Design review of the part built by this model. Coordinates are the model's own, in mm. Face numbers are marked on the shaded views. Coordinates: 2 decimals unless noted, no trailing zeros. Order: outer loops, then holes, each group sorted by start corner. A loop starts at its lowest first (then second) coordinate and runs counter-clockwise, first axis right, second up. Notation, with made-up numbers: M -24,-25.75 L -9,-25.75 A15 cw -9,-21.75 Z; hole C 82,69 d2. An arc over 180 degrees is marked long. Use CSV: the item, a comma, the result in double quotes.
```python
from build123d import *

# Parameters (mm, degrees)
SKETCH1_R           = 9.5
BOSS_EXTRUDE1_DEPTH = 25
SKETCH2_R           = 2.5
CUT_EXTRUDE1_DEPTH  = 15
SKETCH3_R           = 4
CUT_EXTRUDE2_DEPTH  = 20.767397401
CHAMFER1_SIZE       = 2
CUT_EXTRUDE3_REACH  = 34.806
SKETCH13_R          = 1


with BuildPart() as part:
    # Sketch1 → Boss-Extrude1 (new body)
    with BuildSketch(Plane(origin=(0, 0, 0), x_dir=(1, 0, 0), z_dir=(0, 1, 0))):
        with Locations(Location((0, 0, 0), (0, 0, 270))):
            Circle(SKETCH1_R)
    extrude(amount=BOSS_EXTRUDE1_DEPTH)

    # Sketch2 → Cut-Extrude1 (cut)
    with BuildSketch(Plane(origin=(0, 0, 0), x_dir=(1, 0, 0), z_dir=(0, 1, 0))):
        with Locations(Location((0, 0, 0), (0, 0, 270))):
            Circle(SKETCH2_R)
    extrude(amount=CUT_EXTRUDE1_DEPTH, mode=Mode.SUBTRACT)

    # Sketch3 → Cut-Extrude2 (cut, through all)
    with BuildSketch(Plane(origin=(0, 14.5, 0), x_dir=(1, 0, 0), z_dir=(0, 1, 0))):
        with Locations(Location((0, 0, 0), (0, 0, 90))):
            Circle(SKETCH3_R)
    extrude(amount=CUT_EXTRUDE2_DEPTH, mode=Mode.SUBTRACT)

    # Chamfer1
    chamfer1_edges = [part.edges().sort_by_distance(p)[0] for p in [
        (0, 0, -9.5),
        (0, 25, -9.5),
    ]]
    chamfer(chamfer1_edges, length=CHAMFER1_SIZE)

    # Sketch13 → Cut-Extrude3 (cut, up to next)
    with BuildSketch(Plane.XY.offset(9.5), mode=Mode.PRIVATE) as cut_extrude3_sk1:
        with Locations((0, 19)):
            Circle(SKETCH13_R)
    cut_extrude3_tool1 = extrude(cut_extrude3_sk1.sketch, amount=-CUT_EXTRUDE3_REACH, mode=Mode.PRIVATE) & part.part
    # Sketch13 → Cut-Extrude3 (cut, up to next)
    with BuildSketch(Plane.XY.offset(9.5), mode=Mode.PRIVATE) as cut_extrude3_sk2:
        with Locations((0, 7)):
            Circle(SKETCH13_R)
    cut_extrude3_tool2 = extrude(cut_extrude3_sk2.sketch, amount=-CUT_EXTRUDE3_REACH, mode=Mode.PRIVATE) & part.part
    add(cut_extrude3_tool1.solids().sort_by_distance((0, 19, 9.5))[0], mode=Mode.SUBTRACT)
    add(cut_extrude3_tool2.solids().sort_by_distance((0, 7, 9.5))[0], mode=Mode.SUBTRACT)


solid = part.part
```
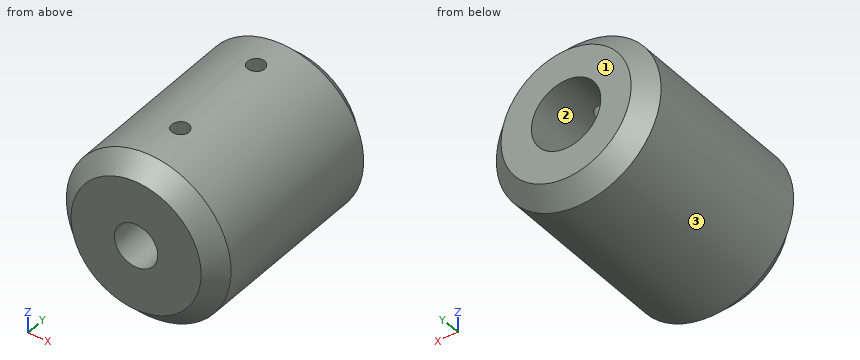
(1) The part is to be moulded in two halves that separate along Z. For the marked faces 1, 2 and 3, say which applies: pulls with the +Z half, pulls with the -Z half, needs draft (parallel to the pull), parting line crosses it, or undercut.
The answers:
face 1,"needs draft"
face 2,"undercut"
face 3,"parting line crosses it"
(2) Add section C-C on y = 21.75. State the section outline as (x, z) points.
The answers:
outline,"C 0,0 d19; hole C 0,0 d8"
(3) Add section D-D on y = 19. State the section outline as (x, z) points.
The answers:
outline,"M -1,3.87 L -1,9.45 A9.5 ccw long 1,9.45 L 1,3.87 A4 cw long Z"
(4) Add section B-B on z = 0. State the section outline as (x, y) points, and give its area (4 significant figures).
The answers:
outline,"M -9.5,2 L -7.5,0 L -2.5,0 L -2.5,14.5 L -4,14.5 L -4,25 L -7.5,25 L -9.5,23 Z; M 2.5,0 L 7.5,0 L 9.5,2 L 9.5,23 L 7.5,25 L 4,25 L 4,14.5 L 2.5,14.5 Z"
area,"310.5 mm2"
(5) Wall thickness on probe 1 along Y at (x, z) = (0, 4.5); probe 2 along X at (y, z) = (3.5, 0); probe 3 along X at (y, z) = (20.75, 0): over which ranges is each line inside the solid? List them lowest first.
The answers:
probe 1,"y = 0 to 6, 8 to 18, 20 to 25"
probe 2,"x = -9.5 to -2.5, 2.5 to 9.5"
probe 3,"x = -9.5 to -4, 4 to 9.5"
(6) Clearance check with flat-ended pins moving along their axes: P1, Ø2, axis at x = -2.5, y = 15, coming from the -Z side; P2, Ø1.6, axis at x = 0, y = 7, coming from the +Z side; P3, Ø1.8, axis at x = 0, y = 19, coming from the +Z side. State where each tip first meets the part, or that it passes through.
The answers:
P1,"stops at z = -9.38"
P2,"stops at z = -2.37"
P3,"stops at z = -3.9"
(7) Add section A-A on x = 0. State the section outline as (y, z) points, and give its area (4 significant figures).
The answers:
outline,"M 0,-7.5 L 2,-9.5 L 23,-9.5 L 25,-7.5 L 25,-4 L 14.5,-4 L 14.5,-2.5 L 0,-2.5 Z; M 0,2.5 L 6,2.5 L 6,9.5 L 2,9.5 L 0,7.5 Z; M 8,2.5 L 14.5,2.5 L 14.5,4 L 18,4 L 18,9.5 L 8,9.5 Z; M 20,4 L 25,4 L 25,7.5 L 23,9.5 L 20,9.5 Z"
area,"285.5 mm2"
